CAD build for the part. Positions are in the model's coordinates, mm. A direction names the side the tool comes from. Coordinates: 2 decimals unless noted, no trailing zeros. Order: outer loops, then holes, each group sorted by start corner. A loop starts at its lowest first (then second) coordinate and runs counter-clockwise, first axis right, second up. Notation, with made-up numbers: (-7.75, -6) - (8.25, -6) arc R11 ccw to (8.25, 10) - close; hole circle Ø7 at (-26.5, 17.5). An arc over 180 degrees is marked (long way). Return JSON: item names as keys, results as strings.
from build123d import *

# Parameters (mm, degrees)
SKETCH_1_R      = 5
EXTRUDE_1_DEPTH = 3
FILLET_1_R      = 0.5
FILLET_2_R      = 1
FILLET_3_R      = 1


with BuildPart() as part:
    # Эскиз1 → Бобышка-Вытянуть1 (new body)
    with BuildSketch(Plane.XY):
        Polygon((39, 19), (-39, 19), (-39, 16), (-52, 16), (-52, 5), (-55, 5), (-55, -5), (-52, -5), (-52, -19), (52, -19), (52, -5), (55, -5), (55, 5), (52, 5), (52, 16), (39, 16), align=None)
        with Locations((-32, -8)):
            Circle(SKETCH_1_R, mode=Mode.SUBTRACT)
        with Locations((-19.2, -8)):
            Circle(SKETCH_1_R, mode=Mode.SUBTRACT)
        with Locations((-6.4, -8)):
            Circle(SKETCH_1_R, mode=Mode.SUBTRACT)
        with Locations((6.4, -8)):
            Circle(SKETCH_1_R, mode=Mode.SUBTRACT)
        with Locations((19.2, -8)):
            Circle(SKETCH_1_R, mode=Mode.SUBTRACT)
        with Locations((32, -8)):
            Circle(SKETCH_1_R, mode=Mode.SUBTRACT)
        with Locations((-32, 10)):
            Circle(SKETCH_1_R, mode=Mode.SUBTRACT)
        with Locations((-19.2, 10)):
            Circle(SKETCH_1_R, mode=Mode.SUBTRACT)
        with Locations((-6.4, 10)):
            Circle(SKETCH_1_R, mode=Mode.SUBTRACT)
        with Locations((6.4, 10)):
            Circle(SKETCH_1_R, mode=Mode.SUBTRACT)
        with Locations((19.2, 10)):
            Circle(SKETCH_1_R, mode=Mode.SUBTRACT)
        with Locations((32, 10)):
            Circle(SKETCH_1_R, mode=Mode.SUBTRACT)
    extrude(amount=EXTRUDE_1_DEPTH)

    # Скругление1
    fillet_1_edges = [part.edges().sort_by_distance(p)[0] for p in [
        (55, 5, 1.5),
        (55, -5, 1.5),
        (-55, -5, 1.5),
        (-55, 5, 1.5),
    ]]
    fillet(fillet_1_edges, radius=FILLET_1_R)

    # Скругление2
    fillet_2_edges = [part.edges().sort_by_distance(p)[0] for p in [
        (-39, 16, 1.5),
        (-39, 19, 1.5),
    ]]
    fillet(fillet_2_edges, radius=FILLET_2_R)

    # Скругление3
    fillet_3_edges = [part.edges().sort_by_distance(p)[0] for p in [
        (39, 19, 1.5),
        (39, 16, 1.5),
    ]]
    fillet(fillet_3_edges, radius=FILLET_3_R)


solid = part.part
Item 1: Band-saw the part on A-A, the plane x = -29. List the corners of the cut face in (y, z).
Findings below:
{"outline": "(-19, 0) - (-12, 0) - (-12, 3) - (-19, 3) - close; (-4, 0) - (6, 0) - (6, 3) - (-4, 3) - close; (14, 0) - (19, 0) - (19, 3) - (14, 3) - close"}
Item 2: Mould opens along X. For faces 1 (the flat face through (53, -5, 1)), 2 (the cylindrical face through (-7.051, -3.043, 1.479)), 3 (the flat face through (-55, 0, 1)) say: released by +X, released by -X, zero draft, split by the parting line, or undercut.
Findings below:
{"face 1": "zero draft", "face 2": "undercut", "face 3": "released by -X"}
Item 3: Which spindle directions (+Z, -Z, +X, -X, +Y, -Y) get a long thin tool onto all of the face, cutting with end or side? Do faces 4 (the flat face through (-52, -12, 1)), 5 (the flat face through (52, 10, 1)), 6 (the cylindrical face through (-19.851, -3.043, 1.479)), 7 (the flat face through (-53, 5, 1)). Say none if no direction does.
Findings below:
{"face 4": "+Z, -Z, -X, -Y", "face 5": "+Z, -Z, +X, +Y", "face 6": "+Z, -Z", "face 7": "+Z, -Z, -X, +Y"}
Item 4: Band-saw the part on D-D, the plane x = 36. List the corners of the cut face in (y, z), then the cut area to 3 significant figures.
Findings below:
{"outline": "(-19, 0) - (-11, 0) - (-11, 3) - (-19, 3) - close; (-5, 0) - (7, 0) - (7, 3) - (-5, 3) - close; (13, 0) - (19, 0) - (19, 3) - (13, 3) - close", "area": "78.0 mm²"}
Item 5: Drop flat-ended pins along their axis: P1, Ø1.2, axis at x = -53, z = 1.5, coming from the +Y side; P2, Ø9, axis at x = -6.4, y = 10, coming from the +Z side. Give the stop position or say it passes through.
Findings below:
{"P1": "stops at y = 5", "P2": "passes through"}
Item 6: Wall check: L1, parallel to Y at x = 6.4, z = 2; L2, parallel to Y at x = 21.5, z = 0.4; L3, parallel to X at y = 17, z = 1.6. Give the ranges that are in metal, low to high. Write a range as [from, to].
Findings below:
{"L1": "y = [-19, -13], [-3, 5], [15, 19]", "L2": "y = [-19, -12.44], [-3.56, 5.56], [14.44, 19]", "L3": "x = [-39, 39]"}
Item 7: Band-saw the part on B-B, the plane y = -8. List the corners of the cut face in (x, z).
Findings below:
{"outline": "(-52, 0) - (-37, 0) - (-37, 3) - (-52, 3) - close; (-27, 0) - (-24.2, 0) - (-24.2, 3) - (-27, 3) - close; (-14.2, 0) - (-11.4, 0) - (-11.4, 3) - (-14.2, 3) - close; (-1.4, 0) - (1.4, 0) - (1.4, 3) - (-1.4, 3) - close; (11.4, 0) - (14.2, 0) - (14.2, 3) - (11.4, 3) - close; (24.2, 0) - (27, 0) - (27, 3) - (24.2, 3) - close; (37, 0) - (52, 0) - (52, 3) - (37, 3) - close"}
Item 8: Band-saw the part on C-C, the plane z = 2.35. Count the separate pieces of the cut face and the enclosed holes in it, then the cut area to 3 significant figures.
Findings below:
{"separate pieces": "1", "enclosed holes": "12", "area": "2,990 mm²"}
